Check sheet for the modelled part. Datum: model origin and axes. Units: mm. Face numbers are marked on the shaded views. A direction names the side the tool comes from. Coordinates: 2 decimals unless noted, no trailing zeros. Loops run counter-clockwise (first coordinate to the right, second up) from the corner with the lowest first, then second, coordinate; pieces in that order, holes last. Notation, with made-up numbers: M 84,52 L 111,52 A25 ccw 111,68 Z; hole C 81,33 d11. An arc over 180 degrees is marked long. Write each question's results on one line, items separated by ' | '. Start each with the question number.
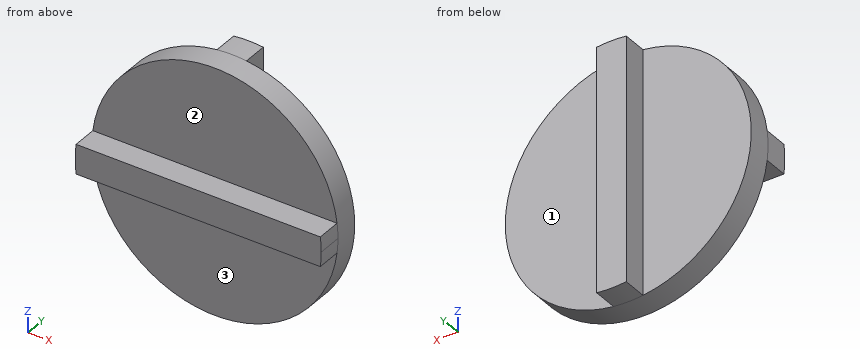
from build123d import *

# Parameters (mm, degrees)
F0_R     = 50
F1_DEPTH = 10
F3_DEPTH = 10
F5_DEPTH = 10


with BuildPart() as f1:
    # F0 (on Front) → F1 (new body)
    with BuildSketch(Plane.XZ):
        Circle(F0_R)
    extrude(amount=F1_DEPTH)

    # F2 (on face) → F3 (join)
    with BuildSketch(Plane.XZ.offset(10)):
        with BuildLine():
            Line((49.638694584, 6), (-49.638694584, 6))
            ThreePointArc((-49.638694584, 6), (-50, 0), (-49.638694584, -6))
            Line((-49.638694584, -6), (49.638694584, -6))
            ThreePointArc((49.638694584, -6), (49.9095919098, -3.0054343115), (50, 0))
            ThreePointArc((50, 0), (49.9095919098, 3.0054343115), (49.638694584, 6))
        make_face()
    extrude(amount=F3_DEPTH)

    # F4 (on Front) → F5 (join)
    with BuildSketch(Plane.XZ):
        with BuildLine():
            Line((6, -49.638694584), (6, 49.638694584))
            ThreePointArc((6, 49.638694584), (0, 50), (-6, 49.638694584))
            Line((-6, 49.638694584), (-6, -49.638694584))
            ThreePointArc((-6, -49.638694584), (0, -50), (6, -49.638694584))
        make_face()
    extrude(amount=-F5_DEPTH)


solid = f1.part
1) Set-up check for the marked faces 1, 2 and 3: record each of +Z, -Z, +X, -X, +Y, -Y from which the full face is reachable in a straight line by a thin tool's end or side.
2) Gauge pin test, flat ends, axial feed: P1, Ø6, axis at x = 13, y = -8.5, coming from the +Z side; P2, Ø22, axis at x = -26.5, z = -21.5, coming from the +Y side; P3, Ø5, axis at x = -24.5, y = -10, coming from the -Z side. Record the tip position at first contact, or that the pin passes through.
3) Thickness scan on probe 1 along Y at (x, z) = (-20, -38.5); probe 2 along Y at (x, z) = (17.5, -3); probe 3 along Z at (x, y) = (40.5, -15.5). Record the ranges inside material, lowest first.
4) Section check C-C (y = -2.75). Enter the section's corners in (x, z), then the cut area to 3 significant figures.
5) Section check A-A (x = 0). Enter the section's corners in (y, z).
6) Section check B-B (z = 15). Enter the section's corners in (x, y).
7) Section check D-D (y = 4.5). Enter the section's corners in (x, z), then the cut area to 3 significant figures.
Return value:
1) face 1: +Z, -Z, +X, +Y | face 2: +Z, +X, -X, -Y | face 3: -Z, +X, -X, -Y
2) P1: stops at z = 48.99 | P2: stops at y = 0 | P3: stops at z = -44.9
3) probe 1: y = -10 to 0 | probe 2: y = -20 to 0 | probe 3: z = -6 to 6
4) outline: C 0,0 d100 | area: 7,850 mm2
5) outline: M -20,-6 L -10,-6 L -10,-50 L 10,-50 L 10,50 L -10,50 L -10,6 L -20,6 Z
6) outline: M -47.7,-10 L 47.7,-10 L 47.7,0 L 6,0 L 6,10 L -6,10 L -6,0 L -47.7,0 Z
7) outline: M -6,-49.64 A50 ccw 6,-49.64 L 6,49.64 A50 ccw -6,49.64 Z | area: 1,200 mm2
